The listing builds one solid part. Answer for the finished solid, in the listing's coordinates (mm). Face numbers are marked on the shaded views. A direction names the side the tool comes from. Coordinates: 2 decimals unless noted, no trailing zeros. Order: outer loops, then holes, each group sorted by start corner. A loop starts at its lowest first (then second) coordinate and runs counter-clockwise, first axis right, second up. Notation, with made-up numbers: (87.25, -29.5) -> (101.25, -29.5) arc R5 ccw to (101.25, -22.5) -> close; hole circle Ø8 at (-17.75, -18.5). An arc over 180 degrees is marked (long way). One line per question, with ' | ' between items.
from build123d import *

# Parameters (mm, degrees)
F1_DEPTH = 73.23845
F3_DEPTH = 57.87031
F4_SIZE  = 5.08
F5_R     = 5.07999
F6_W     = 72.171472013
F6_H     = 40.1722677052


# Not quite as in the source:
# - a fillet or chamfer is up to 0.001 mm smaller than in the source, because OpenCascade refuses the exact size


with BuildPart() as f1:
    # F0 (on Front) → F1 (new body)
    with BuildSketch(Plane.XZ):
        Polygon((0, 59.2983625829), (-118.0220618844, 0), (142.4238681793, 0), align=None)
    extrude(amount=F1_DEPTH)

    # F2 (on face) → F3 (join)
    with BuildSketch(Plane(origin=(0, 0, 0), x_dir=(1, 0, 0), z_dir=(0, 0, -1))):
        Polygon((69.1764354706, 36.619225), (0, 73.23845), (0, 0), align=None)
        Polygon((0, 0), (0, 73.23845), (-63.5601058602, 36.619225), align=None)
    extrude(amount=F3_DEPTH)

    # F4
    f4_edges = [f1.edges().sort_by_distance(p)[0] for p in [
        (34.588218, -18.309613, -57.87031),
        (34.588218, -54.928838, -57.87031),
    ]]
    chamfer(f4_edges, length=F4_SIZE)

    # F5 (radius 5.08 in the source; OpenCascade refuses exactly that, so slightly less here)
    f5_edges = [f1.edges().sort_by_distance(p)[0] for p in [
        (-34.37973, -53.431071, -57.87031),
        (-34.37973, -19.807379, -57.87031),
        (26.559471, -19.807379, -57.87031),
        (26.559471, -53.431071, -57.87031),
    ]]
    fillet(f5_edges, radius=F5_R)

    # F6 (on Front) → F7 (revolve)
    with BuildSketch(Plane.XZ):
        with Locations((-36.0857360065, 20.0861338526)):
            Rectangle(F6_W, F6_H)
    revolve(axis=Axis((-31.7800580476, -18.3096154484, -52.79032), (0.8664808713, 0.4992102759, 0)))


solid = f1.part
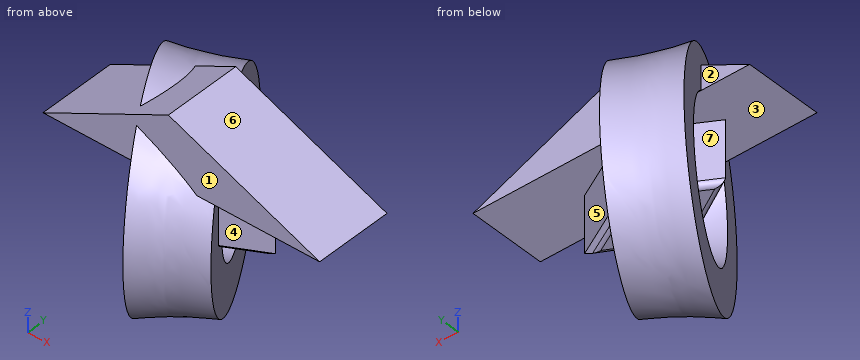
Item 1: For the marked faces 1, 2, 3 and 4, determine the directions among +Z, -Z, +X, -X, +Y, -Y from which every point of the face is accessible in a straight line to the end or side of a thin tool.
Computed values:
face 1: +Z, -Y | face 2: +Z, -Z, -X | face 3: -X | face 4: -Z, +X
Item 2: Determine the mould class of the marked faces 5, 6 and 7 for opening direction Z: pulls with the +Z half, pulls with the -Z half, needs draft (parallel to the pull), parting line crosses it, or undercut.
Computed values:
face 5: needs draft | face 6: pulls with the +Z half | face 7: undercut
Item 3: Section A-A, the plane x = 122 is taken. Give the vertices of the cut face in (y, z), plus the area to 3 significant figures.
Computed values:
outline: (-73.24, 0) -> (0, 0) -> (0, 8.5) -> (-73.24, 8.5) -> close | area: 623 mm^2
Item 4: Each of these flat-tipped pins is pushed along its axis until it touches: pin 1 Ø1 at (y, z) = (-20.5, -97.5) entering from +X; pin 2 Ø1.5 at (x, y) = (-42.5, 47.5) entering from +Z; pin 3 Ø22 at (x, y) = (64.5, -47.5) entering from -Z; pin 4 Ø12 at (x, y) = (0, -80.5) entering from +Z. Where does it stop, or does it pass through?
Computed values:
pin 1: passes through | pin 2: stops at z = 17.22 | pin 3: stops at z = -56.36 | pin 4: stops at z = 18.84
Item 5: Find the intervals of material crossed by L1, parallel to Y at x = 45, z = -39.5; L2, parallel to Z at x = -30, y = 17; L3, parallel to Y at x = -30.5, z = -30, in increasing order.
Computed values:
L1: y = -80.26 to -78.11, -49.42 to -23.82 | L2: z = -141.45 to -97.58, -8 to 35.87 | L3: y = -55.67 to -17.57, 37.62 to 52.94
